Autodesk Inventor part; units mm, degrees
ref_plane "YZ Plane" through (0, 0, 0) normal (1, 0, 0) x (0, 1, 0)
ref_plane "XZ Plane" through (0, 0, 0) normal (0, 1, 0) x (-1, 0, 0)
ref_plane "XY Plane" through (0, 0, 0) normal (0, 0, 1) x (1, 0, 0)
sketch "Sketch1" plane through (0, 0, 0) normal (0, 0, 1) x (1, 0, 0)
  circle A0 centre (0, 0) radius 47.625
  dimension "d0" = 95.25
extrude "Extrusion1" add sketch "Sketch1" along normal blind 3.175
sketch "Sketch3" plane through (0, 0, 3.175) normal (0, 0, 1) x (1, 0, 0)
  line L0 (1.27, 9.525) -> (20.32, 9.525)
  line L1 (20.32, 9.525) -> (20.32, 0)
  line L2 (20.32, 0) -> (1.27, 0)
  line L3 (1.27, 0) -> (1.27, 9.525)
  line L4 (0, 0) -> (0, -11.0035)
  line L5 (-1.27, 9.525) -> (-20.32, 9.525)
  line L6 (-20.32, 9.525) -> (-20.32, 0)
  line L7 (-20.32, 0) -> (-1.27, 0)
  line L8 (-1.27, 0) -> (-1.27, 9.525)
  dimension "d11" = 19.05
  dimension "d12" = 9.525
  dimension "d13" = 1.27
  dimension "d14" = 0
extrude "Extrusion3" add sketch "Sketch3" along normal blind 22.225
sketch "Sketch4" plane through (1.27, 9.525, 3.175) normal (0, 1, 0) x (1, 0, 0)
  circle A0 centre (4.445, -18.415) radius 1.397
  line L0 (19.05, -22.225) -> (0, -22.225)
  circle A1 centre (14.605, -18.415) radius 1.397
  line L1 (9.525, -22.225) -> (9.525, -7.9119)
  line L2 (-1.27, 3.175) -> (-1.27, 8.3959)
  circle A2 centre (-6.985, -18.415) radius 1.397
  circle A3 centre (-17.145, -18.415) radius 1.397
  dimension "d17" = 2.794
  dimension "d18" = 3.81
  dimension "d19" = 2.794
  dimension "d20" = 3.81
  dimension "d21" = 10.16
  dimension "d22" = 5.08
extrude "Extrusion4" cut sketch "Sketch4" against normal through all
sketch "Sketch5" plane through (0, 0, 0) normal (0, 0, -1) x (-1, 0, 0)
  circle A0 centre (12.446, -29.7561) radius 2.3813
  point P0 (0, 0)
  dimension "d25" = 4.7625
  dimension "d26" = 12.446
  dimension "d27" = 29.7561
extrude "Extrusion5" cut sketch "Sketch5" against normal blind 25.4
sketch "Sketch9" plane through (0, 0, 0) normal (0, 0, -1) x (-1, 0, 0)
  line L0 (0, 0) -> (21.4313, 37.12)
  line L1 (0, 0) -> (42.8625, 0) construction
  circle A0 centre (21.4313, 37.12) radius 1.8415
  circle A1 centre (-21.4312, 37.12) radius 1.8415
  circle A2 centre (-42.8625, 0) radius 1.8415
  circle A3 centre (-21.4313, -37.12) radius 1.8415
  circle A4 centre (21.4312, -37.12) radius 1.8415
  circle A5 centre (42.8625, 0) radius 1.8415
  dimension "d44" = 42.8625
  dimension "d45" = 60
  dimension "d46" = 3.683
  dimension "d49" = 360
extrude "Extrusion9" cut sketch "Sketch9" against normal blind 25.4
sketch "Sketch10" plane through (0, 0, 3.175) normal (0, 0, 1) x (1, 0, 0)
  line L0 (0, 0) -> (0, 41.91)
  circle A0 centre (0, 41.91) radius 1.8415
  circle A1 centre (-36.2951, 20.955) radius 1.8415
  circle A2 centre (-36.2951, -20.955) radius 1.8415
  circle A3 centre (0, -41.91) radius 1.8415
  circle A4 centre (36.2951, -20.955) radius 1.8415
  circle A5 centre (36.2951, 20.955) radius 1.8415
  dimension "d53" = 41.91
  dimension "d54" = 3.683
  dimension "d57" = 360
extrude "Extrusion10" cut sketch "Sketch10" against normal blind 25.4
sketch "Sketch11" plane through (0, 0, 3.175) normal (0, 0, 1) x (1, 0, 0)
  line L0 (0, 0) -> (39.3779, 10.5513)
  line L1 (0, 0) -> (40.767, 0) construction
  circle A0 centre (39.3779, 10.5513) radius 2.794
  line L2 (0, 0) -> (0, 16.7096)
  circle A1 centre (39.3779, -10.5513) radius 2.794
  line L3 (0, 0) -> (-40.767, 0) construction
  circle A2 centre (-39.3779, 10.5513) radius 2.794
  circle A3 centre (-39.3779, -10.5513) radius 2.794
  line L4 (0, 0) -> (28.8266, 28.8266)
  line L5 (0, 0) -> (40.767, 0) construction
  circle A4 centre (28.8266, 28.8266) radius 2.794
  circle A5 centre (-28.8266, 28.8266) radius 2.794
  dimension "d61" = 40.767
  dimension "d62" = 15
  dimension "d63" = 5.588
  dimension "d66" = 40.767
  dimension "d67" = 45
  dimension "d68" = 5.588
extrude "Extrusion11" cut sketch "Sketch11" against normal blind 25.4 contours A0 | A1 | A2 | A3
extrude "Extrusion12" cut sketch "Sketch11" against normal blind 25.4 contours A4 | A5
sketch "Sketch12" plane through (0, 0, 3.175) normal (0, 0, 1) x (1, 0, 0)
  circle A0 centre (10.16, -20.32) radius 1.397
  circle A1 centre (10.16, -20.32) radius 4.445
  point P0 (0, 0)
  dimension "d71" = 2.794
  dimension "d72" = 8.89
  dimension "d73" = 20.32
  dimension "d74" = 10.16
extrude "Extrusion13" add sketch "Sketch12" along normal blind 7.62
fillet "Fillet2" radius 3.175 1 edges at (5.715, -20.32, 3.175)
sketch "Sketch13" plane through (0, 0, 3.175) normal (0, 0, 1) x (1, 0, 0)
  circle A0 centre (7.9375, 29.1338) radius 3.3655
  point P0 (0, 0)
  dimension "d79" = 6.731
  dimension "d80" = 29.1338
  dimension "d81" = 7.9375
extrude "Extrusion14" cut sketch "Sketch13" against normal through all
sketch "Sketch16" plane through (0, 0, 3.175) normal (0, 0, 1) x (1, 0, 0)
  circle A0 centre (-2.9972, 33.909) radius 3.3655
  circle A1 centre (-2.9972, 33.909) radius 5.715
  circle A2 centre (7.9375, 29.1338) radius 3.3655
  line L0 (-2.9972, 33.909) -> (7.9375, 29.1338) construction
  point P0 (0, 0)
  dimension "d90" = 6.731
  dimension "d91" = 11.43
  dimension "d92" = 33.909
  dimension "d93" = 2.9972
  dimension "d97" = 11.9319
extrude "Extrusion16" add sketch "Sketch16" along normal blind 3.175 contours A1
fillet "Fillet3" radius 1.27 1 edges at (-8.7122, 33.909, 3.175)
sketch "Sketch18" plane through (0, 0, 3.175) normal (0, 0, 1) x (1, 0, 0)
  arc A0 (0.2617, 40.0872) -> (-1.3949, 40.7077) centre (0, 41.91) ccw construction
  circle A1 centre (0, 41.91) radius 3.81
  point P0 (0, 0)
  dimension "d98" = 7.62
extrude "Extrusion17" cut sketch "Sketch18" along normal through all
fillet "Fillet4" radius 1.27 4 edges at (-3.2657, 39.9475, 3.5916) (1.1725, 38.2849, 3.5916) (0.7956, 38.184, 5.3975) (-3.0478, 39.6238, 5.3975)
sketch "Sketch19" plane through (0, 0, 3.175) normal (0, 0, 1) x (1, 0, 0)
  circle A0 centre (22.86, 16.51) radius 3.81
  circle A1 centre (22.86, 16.51) radius 1.27
  point P0 (0, 0)
  dimension "d102" = 7.62
  dimension "d103" = 2.54
  dimension "d104" = 16.51
  dimension "d105" = 22.86
sketch "Sketch17" plane through (0, 0, 3.175) normal (0, 0, 1) x (1, 0, 0)
  line L0 (-26.0165, 23.6107) -> (-5.4123, 23.6107) construction
  line L1 (-5.4123, 23.6107) -> (-5.4123, 21.8703) construction
  line L2 (-5.4123, 21.8703) -> (-26.0165, 21.8703) construction
  line L3 (-26.0165, 21.8703) -> (-26.0165, 23.6107) construction
extrude "Extrusion18" add sketch "Sketch19" along normal blind 11.684
sketch "Sketch20" plane through (0, 0, 3.175) normal (0, 0, 1) x (1, 0, 0)
  circle A0 centre (-21.4313, 37.12) radius 1.8415
  circle A1 centre (-21.4313, 37.12) radius 3.683
  point P0 (0, 0)
  dimension "d108" = 7.366
extrude "Extrusion19" cut sketch "Sketch20" against normal blind 1.27 contours A0 | A1
pattern_circular "Circular Pattern1" count 6 over 360 about axis through (0, 0, 0) along (0, 0, 1) of "Extrusion19"
fillet "Fillet5" radius 1.524 1 edges at (19.05, 16.51, 3.175)
properties part number "frontServoAttachmentPlate" material "ABS Plastic"
Model file for the job. Use its own axes, mm. A direction names the side the tool comes from. Give positions to 0.01 mm unless a question says otherwise; leave off trailing zeros. Loops run counter-clockwise (first coordinate to the right, second up) from the corner with the lowest first, then second, coordinate; pieces in that order, holes last.
Item 1: Which spindle directions (+Z, -Z, +X, -X, +Y, -Y) get a long thin tool onto all of the face, cutting with end or side? Do faces 4 (the face through (11, 0, 14)), 5 (the face through (-14.646, -30.668, 1.565)), 6 (the face through (-21.91, 40.77, 2.55)). Say none if no direction does.
Check values:
face 4: +Z, +X, -X
face 5: +Z, -Z
face 6: +Z
Item 2: Slice it at D-D (x = 10.16). Write the cut outline in (y, z) (3 decimals).
Check values:
outline: (-46.529, 0) - (26.607, 0) - (26.607, 3.175) - (9.525, 3.175) - (9.525, 25.4) - (0, 25.4) - (0, 3.175) - (-12.7, 3.175) arc R3.175 cw to (-15.875, 6.35) - (-15.875, 10.795) - (-18.923, 10.795) - (-18.923, 3.175) - (-21.717, 3.175) - (-21.717, 10.795) - (-24.765, 10.795) - (-24.765, 6.35) arc R3.175 cw to (-27.94, 3.175) - (-46.529, 3.175) - close; (31.661, 0) - (46.529, 0) - (46.529, 3.175) - (31.661, 3.175) - close
Item 3: Mould opens along Y. For faces 1 (the face through (23, 17, 3.175)), 2 (the face through (-11, 0, 14)), 3 (the face through (-14.543, 4.829, 21.17)) say: +Y half, -Y half, draft (parallel to the pull), parting line (faces both ways), or undercut.
Check values:
face 1: undercut
face 2: -Y half
face 3: draft
Item 4: Drop flat-ended pins along their axis: P1, Ø4, axis at x = 36.3, y = -20.96, coming from the +Z side (3 decimals); P2, Ø3.5, axis at x = 21.43, y = 37.12, coming from the -Z side; P3, Ø12, axis at x = 19.5, z = 20, coming from the +Y side; P4, Ø1, axis at y = 12.5, z = 5, coming from the -X side. Give the stop position or say it passes through.
Check values:
P1: stops at z = 3.175
P2: passes through
P3: stops at y = 20.31
P4: stops at x = 21.38
Item 5: Drill centre lines: line 1 along X through (y, z) = (36, 1.5); line 2 along X through (y, z) = (34, 2); line 3 along X through (y, z) = (0.5, 16.5). Where is each one in solid material? Low to high.
Check values:
line 1: x = -31.18 to -22.89, -19.97 to 19.97, 22.89 to 31.18
line 2: x = -33.35 to -23.39, -19.47 to 19.47, 23.39 to 33.35
line 3: x = -20.32 to -1.27, 1.27 to 20.32
Item 6: Slice it at A-A (x = -29). Write the cut outline in (y, z) (3 decimals).
Check values:
outline: (-37.778, 0) - (26.038, 0) - (26.038, 3.175) - (-37.778, 3.175) - close; (31.615, 0) - (37.778, 0) - (37.778, 3.175) - (31.615, 3.175) - close
Item 7: Slice it at B-B (y = 41.91). Write the cut outline in (x, z) (1 decimal), plus the area to 3 significant figures.
Check values:
outline: (-22.6, 0) - (-1.8, 0) - (-1.8, 3.2) - (-22.6, 3.2) - close; (1.8, 0) - (22.6, 0) - (22.6, 3.2) - (1.8, 3.2) - close
area: 132 mm2
Item 8: Slice it at C-C (y = 16.51). Write the cut outline in (x, z) (3 decimals).
Check values:
outline: (-44.672, 0) - (44.672, 0) - (44.672, 3.175) - (28.194, 3.175) arc R1.524 cw to (26.67, 4.699) - (26.67, 14.859) - (24.13, 14.859) - (24.13, 3.175) - (21.59, 3.175) - (21.59, 14.859) - (19.05, 14.859) - (19.05, 4.699) arc R1.524 cw to (17.526, 3.175) - (-44.672, 3.175) - close
